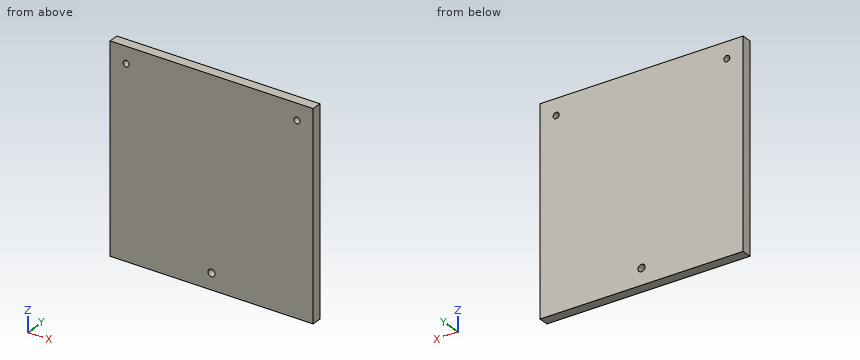
Autodesk Inventor part; units mm, degrees
ref_plane "YZ Plane" through (0, 0, 0) normal (1, 0, 0) x (0, 1, 0)
ref_plane "XZ Plane" through (0, 0, 0) normal (0, 1, 0) x (-1, 0, 0)
ref_plane "XY Plane" through (0, 0, 0) normal (0, 0, 1) x (1, 0, 0)
sketch "Sketch1" plane through (0, 0, 0) normal (0, 1, 0) x (-1, 0, 0)
  line L0 (50, -50) -> (-50, -50)
  line L1 (-50, -50) -> (-50, 50)
  line L2 (-50, 50) -> (50, 50)
  line L3 (50, 50) -> (50, -50)
  line L4 (50, -50) -> (-50, 50) construction
  line L5 (-50, -50) -> (50, 50) construction
  point P0 (0, 0)
  dimension "d0" = 100
  dimension "d1" = 100
extrude "Extrusion1" add sketch "Sketch1" along normal blind 5
sketch "Sketch2" plane through (0, 5, 0) normal (0, 1, 0) x (1, 0, 0)
  circle A0 centre (42, 0) radius 4
  circle A1 centre (42, -42) radius 1.5
  circle A2 centre (-42, -42) radius 1.5
  circle A3 centre (-42, 0) radius 4
  circle A4 centre (0, 42) radius 1.75
  line L0 (-50, -50) -> (-50, 50)
  line L1 (50, 50) -> (-50, 50)
  line L2 (-50, -50) -> (50, -50)
  line L3 (50, 50) -> (50, -50)
  point P0 (0, 0)
  dimension "d5" = 8
  dimension "d6" = 3
  dimension "d7" = 3
  dimension "d8" = 8
  dimension "d9" = 3.5
  dimension "d12" = 8
  dimension "d13" = 8
  dimension "d14" = 8
  dimension "d15" = 8
  dimension "d16" = 8
  dimension "d17" = 8
  dimension "d22" = 50
  dimension "d23" = 8
extrude "Extrusion2" cut sketch "Sketch2" against normal blind 5 contours A1 | A2 | A4
properties part number "print"
Can you work these out from the model? Positions are in its coordinate system, mm. Round coordinates to 2 decimals unless told otherwise and drop trailing zeros. Loops run counter-clockwise (first coordinate to the right, second up) from the corner with the lowest first, then second, coordinate; pieces in that order, holes last. Notation, with made-up numbers: M -2,-16 L 9,-16 A14 cw 9,-4 Z; hole C 74.5,77.5 d10. An arc over 180 degrees is marked long. Answer in a Markdown table with one row per item.
1. I'm going to push a flat-ended pin straight in: pin 1 Ø4 at (x, z) = (42, 42) entering from -Y. Where does the tip first touch, or does it pass through?
Established:
| item | result |
|---|---|
| pin 1 | y = 0 |
2. If we section it at C-C, the plane z = -42: Please give me the cut outline in (x, y), plus the area to 4 significant figures.
Established:
| item | result |
|---|---|
| outline | M -50,0 L -1.75,0 L -1.75,5 L -50,5 Z; M 1.75,0 L 50,0 L 50,5 L 1.75,5 Z |
| area | 482.5 mm² |
3. Please list where these lines run through material, in increasing order: line 1 (X direction, y = 2.65, z = 42); line 2 (Z direction, x = 0, y = 3.05); line 3 (Z direction, x = -42, y = 3.1). Write a range as from..to.
Established:
| item | result |
|---|---|
| line 1 | -50..-43.5, -40.5..40.5, 43.5..50 |
| line 2 | -50..-43.75, -40.25..50 |
| line 3 | -50..40.5, 43.5..50 |
4. If we section it at A-A, the plane z = 42: Please give me the cut outline in (x, y).
Established:
| item | result |
|---|---|
| outline | M -50,0 L -43.5,0 L -43.5,5 L -50,5 Z; M -40.5,0 L 40.5,0 L 40.5,5 L -40.5,5 Z; M 43.5,0 L 50,0 L 50,5 L 43.5,5 Z |
5. If we section it at B-B, the plane x = 42: Please give me the cut outline in (y, z), plus the area to 3 significant figures.
Established:
| item | result |
|---|---|
| outline | M 0,-50 L 5,-50 L 5,40.5 L 0,40.5 Z; M 0,43.5 L 5,43.5 L 5,50 L 0,50 Z |
| area | 485 mm² |
